For this review, take the finished solid that the model builds, in its own axes (mm). Round coordinates to 2 decimals unless told otherwise and drop trailing zeros. Loops run counter-clockwise (first coordinate to the right, second up) from the corner with the lowest first, then second, coordinate; pieces in that order, holes last. Notation, with made-up numbers: (27.25, 72) -> (71.25, 72) arc R25 cw to (71.25, 102) -> close; hole circle Ø10 at (-31, -19). An arc over 180 degrees is marked (long way). Write each question's results on one line, items separated by ' | '.
```python
from build123d import *

# Parameters (mm, degrees)
IZIM1_W                     = 50
IZIM1_H                     = 50
IZIM1_H_2                   = 45
IZIM1_W_2                   = 45
Y_KSEKLIK_EKSTR_ZYON2_DEPTH = 5
IZIM2_R                     = 3
Y_KSEKLIK_EKSTR_ZYON3_DEPTH = 15
Y_KSEKLIK_EKSTR_ZYON4_DEPTH = 6
IZIM4_W                     = 15
IZIM4_H                     = 5
IZIM4_W_2                   = 5
IZIM4_H_2                   = 15
Y_KSEKLIK_EKSTR_ZYON5_DEPTH = 20
IZIM5_R                     = 2
KES_EKSTR_ZYON1_DEPTH       = 132.1
IZIM6_R                     = 2
KES_EKSTR_ZYON2_DEPTH       = 169.6
IZIM7_W                     = 393.876615126
IZIM7_H                     = 303.042246628
KES_EKSTR_ZYON3_DEPTH       = 26
KES_EKSTR_ZYON4_DEPTH       = 7


with BuildPart() as part:
    # Çizim1 → Yükseklik-Ekstrüzyon2 (new body)
    with BuildSketch(Plane.XY):
        Polygon((-35, -128.6), (-35, -116.312863708), (-52.209867178, -116.312863708), align=None)
        Polygon((-35, -116.312863708), (-148.890132822, -35), (-148.890132822, -47.287136292), (-52.209867178, -116.312863708), align=None)
        Polygon((-25, -35), (-35, -35), (-35, -116.312863708), (-35, -128.6), (35, -128.6), (35, -116.312863708), (35, -35), (25, -35), (25, -80), (25, -108.6), (-25, -108.6), (-25, -80), align=None)
        Polygon((-148.890132822, -47.287136292), (-166.1, -35), (-166.1, -128.6), (-35, -128.6), (-52.209867178, -116.312863708), (-148.890132822, -116.312863708), align=None)
        Polygon((-148.890132822, -35), (-166.1, -35), (-148.890132822, -47.287136292), align=None)
        Polygon((-35, 25), (-35, 35), (-148.890132822, 35), (-166.1, 35), (-166.1, -35), (-148.890132822, -35), (-35, -35), (-35, -25), (-80, -25), (-146.1, -25), (-146.1, 25), (-80, 25), align=None)
        Polygon((-25, 35), (-35, 35), (-35, 25), (-35, -25), (-35, -35), (-25, -35), (25, -35), (35, -35), (35, -25), (35, 25), (35, 35), (25, 35), align=None)
        Rectangle(IZIM1_W, IZIM1_H, mode=Mode.SUBTRACT)
        with Locations((0, -57.5)):
            Rectangle(IZIM1_W, IZIM1_H_2)
        Rectangle(IZIM1_W, IZIM1_H)
        with Locations((-57.5, 0)):
            Rectangle(IZIM1_W_2, IZIM1_H)
        with Locations((57.5, 0)):
            Rectangle(IZIM1_W_2, IZIM1_H)
        Polygon((148.890132822, 35), (35, 35), (35, 25), (80, 25), (146.1, 25), (146.1, -25), (80, -25), (35, -25), (35, -35), (148.890132822, -35), (166.1, -35), (166.1, 35), align=None)
        Polygon((148.890132822, -47.287136292), (148.890132822, -35), (35, -116.312863708), (52.209867178, -116.312863708), align=None)
        Polygon((148.890132822, -47.287136292), (166.1, -35), (148.890132822, -35), align=None)
        Polygon((166.1, -128.6), (166.1, -35), (148.890132822, -47.287136292), (148.890132822, -116.312863708), (52.209867178, -116.312863708), (35, -128.6), align=None)
        Polygon((52.209867178, -116.312863708), (35, -116.312863708), (35, -128.6), align=None)
        Polygon((52.209867178, 116.312863708), (35, 116.312863708), (148.890132822, 35), (148.890132822, 47.287136292), align=None)
        Polygon((148.890132822, 47.287136292), (148.890132822, 35), (166.1, 35), align=None)
        Polygon((166.1, 128.6), (35, 128.6), (52.209867178, 116.312863708), (148.890132822, 116.312863708), (148.890132822, 47.287136292), (166.1, 35), align=None)
        Polygon((52.209867178, 116.312863708), (35, 128.6), (35, 116.312863708), align=None)
        Polygon((35, 128.6), (-35, 128.6), (-35, 116.312863708), (-35, 35), (-25, 35), (-25, 80), (-25, 108.6), (25, 108.6), (25, 80), (25, 35), (35, 35), (35, 116.312863708), align=None)
        with Locations((0, 57.5)):
            Rectangle(IZIM1_W, IZIM1_H_2)
        Polygon((-35, 116.312863708), (-35, 128.6), (-52.209867178, 116.312863708), align=None)
        Polygon((-35, 116.312863708), (-52.209867178, 116.312863708), (-148.890132822, 47.287136292), (-148.890132822, 35), align=None)
        Polygon((-52.209867178, 116.312863708), (-35, 128.6), (-166.1, 128.6), (-166.1, 35), (-148.890132822, 47.287136292), (-148.890132822, 116.312863708), align=None)
        Polygon((-148.890132822, 35), (-148.890132822, 47.287136292), (-166.1, 35), align=None)
    extrude(amount=-Y_KSEKLIK_EKSTR_ZYON2_DEPTH)

    # Çizim2 → Yükseklik-Ekstrüzyon3 (add)
    with BuildSketch(Plane(origin=(0, 0, -5), x_dir=(-1, 0, 0), z_dir=(0, 0, -1))):
        Circle(IZIM2_R)
    extrude(amount=Y_KSEKLIK_EKSTR_ZYON3_DEPTH)

    # Çizim3 → Yükseklik-Ekstrüzyon4 (add)
    with BuildSketch(Plane.XY):
        Polygon((161.1, 123.6), (161.1, 25), (166.1, 25), (166.1, 128.6), (-166.1, 128.6), (-166.1, -128.6), (166.1, -128.6), (166.1, -25), (161.1, -25), (161.1, -123.6), (-161.1, -123.6), (-161.1, 123.6), align=None)
    extrude(amount=Y_KSEKLIK_EKSTR_ZYON4_DEPTH)

    # Çizim4 → Yükseklik-Ekstrüzyon5 (add)
    with BuildSketch(Plane(origin=(0, 0, -5), x_dir=(-1, 0, 0), z_dir=(0, 0, -1))):
        with Locations((-60, 0)):
            Rectangle(IZIM4_W, IZIM4_H)
        with Locations((0, -60)):
            Rectangle(IZIM4_W_2, IZIM4_H_2)
    extrude(amount=Y_KSEKLIK_EKSTR_ZYON5_DEPTH)

    # Çizim5 → Kes-Ekstrüzyon1 (cut, through all)
    with BuildSketch(Plane.XZ.offset(2.5)):
        with Locations((60, -10)):
            Circle(IZIM5_R)
        with Locations((60, -19)):
            Circle(IZIM5_R)
    extrude(amount=-KES_EKSTR_ZYON1_DEPTH, mode=Mode.SUBTRACT)

    # Çizim6 → Kes-Ekstrüzyon2 (cut, through all)
    with BuildSketch(Plane(origin=(2.5, 0, 0), x_dir=(0, 0, -1), z_dir=(1, 0, 0))):
        with Locations((10, -60)):
            Circle(IZIM6_R)
        with Locations((19, -60)):
            Circle(IZIM6_R)
    extrude(amount=-KES_EKSTR_ZYON2_DEPTH, mode=Mode.SUBTRACT)

    # Çizim7 → Kes-Ekstrüzyon3 (cut, through all)
    with BuildSketch(Plane.XY):
        with Locations((1.174582351, -1.957637252)):
            Rectangle(IZIM7_W, IZIM7_H)
    extrude(amount=-KES_EKSTR_ZYON3_DEPTH, mode=Mode.SUBTRACT)

    # Çizim8 → Kes-Ekstrüzyon4 (cut, through all)
    with BuildSketch(Plane.XY.offset(6)):
        Polygon((161.1, 25), (163.1, 25), (163.1, 125.6), (-163.1, 125.6), (-163.1, -125.6), (163.1, -125.6), (163.1, -25), (161.1, -25), (161.1, -123.6), (-161.1, -123.6), (-161.1, 123.6), (161.1, 123.6), align=None)
    extrude(amount=-KES_EKSTR_ZYON4_DEPTH, mode=Mode.SUBTRACT)


solid = part.part
```
1. To check wall thickness, follow probe 1 along X at (y, z) = (-42, 4.95); probe 2 along Y at (x, z) = (122, 1.85); probe 3 along X at (y, z) = (-7, 1.7). State the ranges of each line that lie inside material, in increasing order.
Values found:
probe 1: x = -166.1 to -163.1, 163.1 to 166.1 | probe 2: y = -128.6 to -125.6, 125.6 to 128.6 | probe 3: x = -166.1 to -163.1
2. Consider section A-A (y = -45). State the section outline as (x, z) points, plus the area to 3 significant figures.
Values found:
outline: (-166.1, 0) -> (-163.1, 0) -> (-163.1, 6) -> (-166.1, 6) -> close; (163.1, 0) -> (166.1, 0) -> (166.1, 6) -> (163.1, 6) -> close | area: 36.0 mm2
3. Consider section B-B (x = 45). State the section outline as (y, z) points, plus the area to 3 significant figures.
Values found:
outline: (-128.6, 0) -> (-125.6, 0) -> (-125.6, 6) -> (-128.6, 6) -> close; (125.6, 0) -> (128.6, 0) -> (128.6, 6) -> (125.6, 6) -> close | area: 36.0 mm2
4. Consider section C-C (z = 3.85). State the section outline as (x, y) points, plus the area to 3 significant figures.
Values found:
outline: (-166.1, -128.6) -> (166.1, -128.6) -> (166.1, -25) -> (163.1, -25) -> (163.1, -125.6) -> (-163.1, -125.6) -> (-163.1, 125.6) -> (163.1, 125.6) -> (163.1, 25) -> (166.1, 25) -> (166.1, 128.6) -> (-166.1, 128.6) -> close | area: 3,350 mm2
